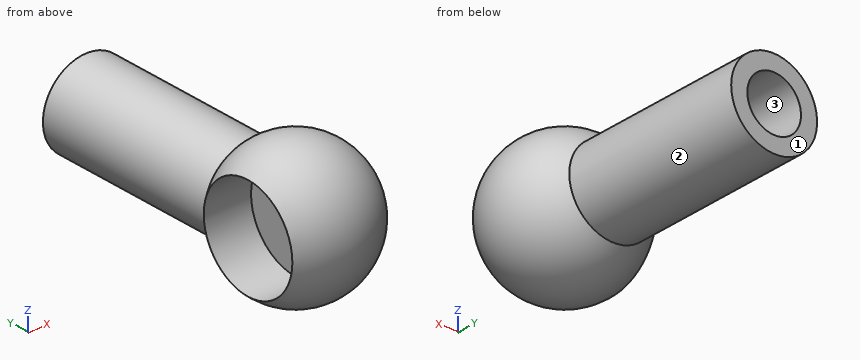
Autodesk Inventor part; units mm, degrees
ref_plane "YZ Plane" through (0, 0, 0) normal (1, 0, 0) x (0, 1, 0)
ref_plane "XZ Plane" through (0, 0, 0) normal (0, 1, 0) x (-1, 0, 0)
ref_plane "XY Plane" through (0, 0, 0) normal (0, 0, 1) x (1, 0, 0)
sketch "스케치1" plane through (0, 0, 0) normal (0, 0, 1) x (1, 0, 0)
  circle A0 centre (0, 0) radius 6.4
  line L0 (0, 6.4) -> (0, -6.4)
  dimension "d0" = 12.8
sketch "스케치1 outline for SR sphere" plane through (0, 0, 0) normal (0, 0, 1) x (1, 0, 0)
  line L0 (0, 6.4) -> (0, -6.4)
  arc A0 (0, -6.4) -> (0, 6.4) centre (0, 0) ccw
revolve "SR sphere" add sketch "스케치1 outline for SR sphere" angle 360 about axis through (0, 6.4, 0) along (0, -1, 0)
sketch "e" plane through (0, 0, 0) normal (1, 0, 0) x (0, 1, 0)
  circle A0 centre (0, 0) radius 4.647459
sketch "e outline for e hole" plane through (0, 0, 0) normal (1, 0, 0) x (0, 1, 0)
  circle A0 centre (0, 0) radius 4.647459
extrude "e hole" cut sketch "e outline for e hole" against normal blind 6.4
sketch "스케치6" plane through (0, 0, 0) normal (0, 0, 1) x (1, 0, 0)
  arc A0 (-4.400128, -4.647459) -> (-4.400128, 4.647459) centre (0, 0) ccw
  line L0 (4.001417, 4.994864) -> (4.001417, 21.987002)
  line L1 (4.001417, 21.987002) -> (2.501417, 21.987002)
  line L2 (2.501417, 21.987002) -> (2.501417, 5.890918)
  line L3 (0.001417, -6.4) -> (0.001417, 19.355985)
  line L4 (10.301781, -0.012998) -> (-6.695287, -0.012998)
  line L5 (4.001417, 4.994864) -> (2.501417, 5.890918)
  point P0 (3.251417, 21.987002)
  dimension "d4" = 1.5
  dimension "d5" = 4
  dimension "d6" = 22
sketch "스케치6 outline for h, g 고려 회전" plane through (0, 0, 0) normal (0, 0, 1) x (1, 0, 0)
  line L0 (4.001417, 21.987002) -> (2.501417, 21.987002)
  line L1 (4.001417, 4.994864) -> (4.001417, 21.987002)
  arc A0 (2.501417, 5.890918) -> (4.001417, 4.994864) centre (0, 0) cw
  line L2 (2.501417, 21.987002) -> (2.501417, 5.890918)
revolve "h, g 고려 회전" add sketch "스케치6 outline for h, g 고려 회전" angle 360 about axis through (0.001417, -6.4, 0) along (0, 1, 0)
properties part number "Ball Joint_bot"
Check sheet for the modelled part. Datum: model origin and axes. Units: mm. Face numbers are marked on the shaded views. Round coordinates to 2 decimals unless told otherwise and drop trailing zeros. Write each loop counter-clockwise with the first axis right and the second up, starting at its lowest first coordinate (ties: lowest second). Pieces come first, ordered by that corner, then holes. Notation, with made-up numbers: M 56,72.5 L 97,72.5 A20 ccw 97,110.5 Z; hole C -27.75,-40 d3. An arc over 180 degrees is marked long. Write item = value, one per line. Start each with the question number.
1. Section check B-B, the plane z = 0.75. Record the cut outline in (x, y).
2. Section check D-D, the plane y = 0. Record the cut outline in (x, z).
3. Release check for a two-part mould opening along X. For the marked faces 1, 2 and 3 record: pulls with the +X half, pulls with the -X half, needs draft (parallel to the pull), parting line crosses it, or undercut.
4. Section check C-C, the plane x = 1.5. Record the cut outline in (y, z), then the cut area to 3 significant figures.
5. Gauge pin test, flat ends, axial feed: pin 1 (4 mm diameter, centred on x = 5, z = 2.5, fed in from +Y); pin 2 (1.5 mm diameter, centred on y = 7, z = 3.5, fed in from +X); pin 3 (3 mm diameter, centred on y = 16, z = -2.5, fed in from +X); pin 4 (6 mm diameter, centred on x = 1.5, y = 10, fed in from -Z). Record the tip position at first contact, or that the pin passes through.
6. Scan lines: line 1 (X direction, y = 21.25, z = 1.5); line 2 (Y direction, x = -1.55, z = 0); line 3 (Z direction, x = -4, y = 0.5). Record each from-to range of solid material in increasing order. Write a range as [from, to].
7. Section check A-A, the plane y = 20. Record the cut outline in (x, z).
Results found:
q1.outline = M -4.4,-4.59 A6.36 ccw long 3.93,4.99 L 3.93,21.99 L 2.39,21.99 L 2.39,5.89 A6.36 ccw -2.38,5.89 L -2.38,21.99 L -3.93,21.99 L -3.93,5 A6.36 ccw -4.4,4.59 L 0,4.59 L 0,-4.59 Z
q2.outline = M -4.4,-4.65 A6.4 ccw long -4.4,4.65 L 0,4.65 L 0,-4.65 Z
q3.face_1 = needs draft
q3.face_2 = parting line crosses it
q3.face_3 = undercut
q4.outline = M 5,-3.71 L 21.99,-3.71 L 21.99,-2 L 5.89,-2 A6.22 ccw 5.89,2 L 21.99,2 L 21.99,3.71 L 5,3.71 A6.22 ccw long Z
q4.area = 178 mm^2
q5.pin_1 = 21.99
q5.pin_2 = 2.91
q5.pin_3 = 3.87
q5.pin_4 = -4
q6.line_1 = [-3.71, -2], [2, 3.71]
q6.line_2 = [-6.21, -4.65], [4.65, 6.21]
q6.line_3 = [-4.97, -4.62], [4.62, 4.97]
q7.outline = C 0,0 d8; hole C 0,0 d5
